```python
from build123d import *

# Parameters (mm, degrees)
F0_R     = 6.35
F1_DEPTH = 25.4


# Not quite as in the source:
# - a feature names something its author has since deleted; it is built from what else it names


with BuildPart() as f1:
    # F0 (on Right) → F1 (new body)
    with BuildSketch(Plane.YZ):
        with BuildLine():
            ThreePointArc((12.4942827194, 13.5984018078), (12.6484661231, 14.7320631111), (12.7, 15.875))
            ThreePointArc((12.7, 15.875), (-1.1429368889, 28.5234661231), (-12.4942827194, 13.5984018078))
            ThreePointArc((-12.4942827194, 13.5984018078), (0, 3.175), (12.4942827194, 13.5984018078))
        make_face()
        with Locations((0, 15.875)):
            Circle(F0_R, mode=Mode.SUBTRACT)
        with BuildLine():
            ThreePointArc((12.4942827194, -13.5984018078), (0, -3.175), (-12.4942827194, -13.5984018078))
            ThreePointArc((-12.4942827194, -13.5984018078), (-1.1429368889, -28.5234661231), (12.7, -15.875))
            ThreePointArc((12.7, -15.875), (12.6484661231, -14.7320631111), (12.4942827194, -13.5984018078))
        make_face()
        with Locations((0, -15.875)):
            Circle(F0_R, mode=Mode.SUBTRACT)
        with BuildLine():
            ThreePointArc((12.4942827194, 13.5984018078), (0, 3.175), (-12.4942827194, 13.5984018078))
            ThreePointArc((-12.4942827194, 13.5984018078), (-11.5006568446, 0), (-12.4942827194, -13.5984018078))
            ThreePointArc((-12.4942827194, -13.5984018078), (0, -3.175), (12.4942827194, -13.5984018078))
            ThreePointArc((12.4942827194, -13.5984018078), (11.5006568446, 0), (12.4942827194, 13.5984018078))
        make_face()
    extrude(amount=F1_DEPTH)


solid = f1.part
```
Design review of the part built by this model. Coordinates are the model's own, in mm. Give positions to 0.01 mm unless a question says otherwise; leave off trailing zeros. Write each loop counter-clockwise with the first axis right and the second up, starting at its lowest first coordinate (ties: lowest second). Pieces come first, ordered by that corner, then holes. Notation, with made-up numbers: (38, 40) - (69, 40) arc R32 cw to (69, 70) - close; hole circle Ø11 at (-9, 69.5). An arc over 180 degrees is marked (long way). Return JSON: item names as keys, results as strings. Group by question number.
(1) Mouldability with a two-part tool opening along Y and no side actions: class faces 1 (the cylindrical face through (12.5, 11.5, -0.2)), 2 (the cylindrical face through (12.522, -1.377, -22.074)), 3 (the flat face through (0, 0, 0)) as +Y half, -Y half, draft (parallel to the pull), parting line (faces both ways), or undercut.
(2) We need section C-C, the plane x = 20.25. Give the boundary of the cut face in (y, z) (3 decimals).
(3) We need section A-A, the plane y = 0. Give the boundary of the cut face in (x, z) (3 decimals), then the cut area to 3 significant figures.
(4) We need section B-B, the plane z = -20. Give the boundary of the cut face in (x, y).
(5) We need section D-D, the plane y = -5. Give the boundary of the cut face in (x, z).
(6) To check wall thickness, follow probe 1 along Z at (x, y) = (16.75, 0) (3 decimals); probe 2 along Z at (x, y) = (10.5, -5.5); probe 3 along Y at (x, z) = (13.25, -12). State the ranges of each line that lie inside material, in increasing order.
(7) Insertion check: pin 1 (12 mm diameter, centred on x = 22.5, z = 6, fed in from -Y); pin 2 (1 mm diameter, centred on x = 20, y = 10, fed in from -Z); pin 3 (11.5 mm diameter, centred on y = 0, z = 15.875, fed in from -X); pin 4 (3 mm diameter, centred on x = 6.5, y = -10, fed in from +Z). Each pin has a flat end and moves straight along its axis. Give the tip position at first contact, or say it passes through.
Reported:
{
 "1": {"face 1": "+Y half", "face 2": "undercut", "face 3": "draft"},
 "2": {"outline": "(-12.494, -13.598) arc R12.7 ccw (long way) to (12.494, -13.598) arc R93.548 cw to (12.494, 13.598) arc R12.7 ccw (long way) to (-12.494, 13.598) arc R93.548 cw to start; hole circle Ø12.7 at (0, -15.875); hole circle Ø12.7 at (0, 15.875)"},
 "3": {"outline": "(0, -28.575) - (25.4, -28.575) - (25.4, -22.225) - (0, -22.225) - close; (0, -9.525) - (25.4, -9.525) - (25.4, 9.525) - (0, 9.525) - close; (0, 22.225) - (25.4, 22.225) - (25.4, 28.575) - (0, 28.575) - close", "area": "806 mm2"},
 "4": {"outline": "(0, -12.01) - (25.4, -12.01) - (25.4, -4.83) - (0, -4.83) - close; (0, 4.83) - (25.4, 4.83) - (25.4, 12.01) - (0, 12.01) - close"},
 "5": {"outline": "(0, -27.55) - (25.4, -27.55) - (25.4, -19.79) - (0, -19.79) - close; (0, -11.96) - (25.4, -11.96) - (25.4, 11.96) - (0, 11.96) - close; (0, 19.79) - (25.4, 19.79) - (25.4, 27.55) - (0, 27.55) - close"},
 "6": {"probe 1": "z = -28.575 to -22.225, -9.525 to 9.525, 22.225 to 28.575", "probe 2": "z = -27.32 to -19.05, -12.7 to 12.7, 19.05 to 27.32", "probe 3": "y = -12.27 to -5.03, 5.03 to 12.27"},
 "7": {"pin 1": "stops at y = -12.27", "pin 2": "stops at z = -24.3", "pin 3": "passes through", "pin 4": "stops at z = 25.31"}
}
